Here's how the part is built. I have some questions about the finished solid (model axes, mm). Face numbers are marked on the shaded views. A direction names the side the tool comes from. Give positions to 0.01 mm unless a question says otherwise; leave off trailing zeros. Loops run counter-clockwise (first coordinate to the right, second up) from the corner with the lowest first, then second, coordinate; pieces in that order, holes last.
Q1. I'm going to push a flat-ended pin straight in: P1, Ø8.5, axis at x = 23.65, z = -10, coming from the +Y side. Where does the tip first touch, or does it pass through?
Q2. Thinking about a two-plate mould opening in X: for the marked faces 1, 2 and 3, which applies, pulls with the +X half, pulls with the -X half, needs draft (parallel to the pull), parting line crosses it, or undercut?
Q3. For the marked faces 4 and 5, which set-ups out of +Z, -Z, +X, -X, +Y, -Y let a thin tool reach every point of the face, with its end or its side?
Q4. Suppose I cut it at B-B (y = 7.5). List the corners of the cut face in (x, z) for me, and give its area (3 significant figures).
Q5. I need wall thicknesses on probe 1 along X at (y, z) = (3.75, -35); probe 2 along Z at (x, y) = (56, 3.75); probe 3 along Z at (x, y) = (23.65, 5.5). Which ranges of each line are inside material? Lowest first, please.
Q6. Suppose I cut it at A-A (z = -39). List the corners of the cut face in (x, y) for me.
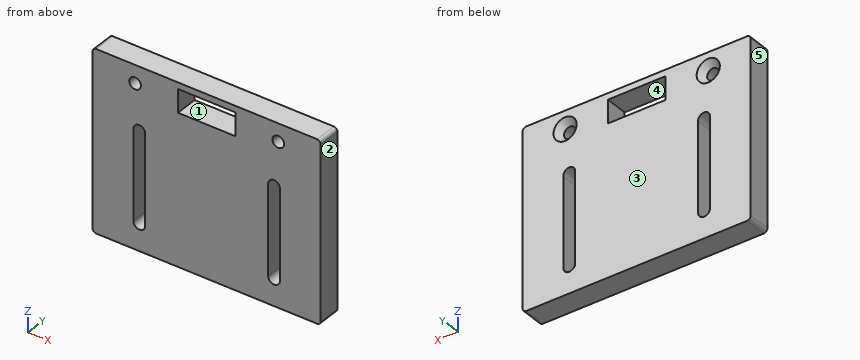
```python
from build123d import *

# Parameters (mm, degrees)
SKETCH1_W                                        = 127
SKETCH1_H                                        = 100
BOSS_EXTRUDE1_DEPTH                              = 12.7
CUT_EXTRUDE1_DEPTH                               = 12.7
CUT_EXTRUDE2_DEPTH                               = 163.142807426
FILLET1_R                                        = 2
CSK_FOR_1_4_FLAT_HEAD_MACHINE_SCREW1_D           = 6.5278
CSK_FOR_1_4_FLAT_HEAD_MACHINE_SCREW1_CSINK_D     = 12.8778
CSK_FOR_1_4_FLAT_HEAD_MACHINE_SCREW1_CSINK_ANGLE = 82


with BuildPart() as part:
    # Sketch1 → Boss-Extrude1 (new body)
    with BuildSketch(Plane(origin=(0, 0, 0), x_dir=(1, 0, 0), z_dir=(0, 1, 0))):
        with Locations((63.5, 50)):
            Rectangle(SKETCH1_W, SKETCH1_H)
    extrude(amount=BOSS_EXTRUDE1_DEPTH)

    # Sketch2 → Cut-Extrude1 (cut)
    with BuildSketch(Plane(origin=(0, 12.7, 0), x_dir=(1, 0, 0), z_dir=(0, 1, 0))):
        Polygon((47.53, 10), (47.53, 16.45), (79.48, 16.45), (79.48, 10), (79.48, 3.55), (47.53, 3.55), align=None)
    extrude(amount=-CUT_EXTRUDE1_DEPTH, mode=Mode.SUBTRACT)

    # Sketch6 → Cut-Extrude2 (cut, through all)
    with BuildSketch(Plane(origin=(0, 12.7, 0), x_dir=(1, 0, 0), z_dir=(0, 1, 0))):
        with BuildLine():
            Line((22.690847092, 35), (22.690847092, 85))
            ThreePointArc((22.690847092, 85), (25.990847092, 88.3), (29.290847092, 85))
            Line((29.290847092, 85), (29.290847092, 35))
            ThreePointArc((29.290847092, 35), (25.990847092, 31.7), (22.690847092, 35))
        make_face()
        with BuildLine():
            Line((97.720847092, 35.000004619), (97.720847092, 84.999995381))
            ThreePointArc((97.720847092, 84.999995381), (100.881876157, 88.297072501), (104.30914268, 85.2776907))
            Line((104.30914268, 85.2776907), (104.30914268, 35.2776907))
            ThreePointArc((104.30914268, 35.2776907), (101.159813412, 31.702927304), (97.720847092, 35.000004619))
        make_face()
    extrude(amount=-CUT_EXTRUDE2_DEPTH, mode=Mode.SUBTRACT)

    # Fillet1
    fillet1_edges = [part.edges().sort_by_distance(p)[0] for p in [
        (0, 6.35, -100),
        (127, 6.35, -100),
        (127, 6.35, 0),
        (0, 6.35, 0),
    ]]
    fillet(fillet1_edges, radius=FILLET1_R)

    # CSK for 1/4 Flat Head Machine Screw1 (through all)
    with Locations(Plane(origin=(23.65, 12.7, -9.996892397), x_dir=(0, 0, 1), z_dir=(0, 1, 0))):
        with Locations((0, 0), (0, 79.7)):
            CounterSinkHole(CSK_FOR_1_4_FLAT_HEAD_MACHINE_SCREW1_D / 2, CSK_FOR_1_4_FLAT_HEAD_MACHINE_SCREW1_CSINK_D / 2, counter_sink_angle=CSK_FOR_1_4_FLAT_HEAD_MACHINE_SCREW1_CSINK_ANGLE)


solid = part.part
```
Solutions:
1. P1: stops at y = 10.19
2. face 1: undercut
2. face 2: pulls with the +X half
2. face 3: needs draft
3. face 4: +Y, -Y
3. face 5: +Z, -Z, -X, +Y, -Y
4. outline: (0, -98) arc R2 ccw to (2, -100) - (125, -100) arc R2 ccw to (127, -98) - (127, -2) arc R2 ccw to (125, 0) - (2, 0) arc R2 ccw to (0, -2) - close; hole circle Ø6.53 at (23.65, -10); hole (22.69, -85) arc R3.3 ccw to (29.29, -85) - (29.29, -35) arc R3.3 ccw to (22.69, -35) - close; hole (47.53, -16.45) - (79.48, -16.45) - (79.48, -3.55) - (47.53, -3.55) - close; hole (97.72, -85) arc R3.3 ccw to (104.31, -85.28) - (104.31, -35.28) arc R3.3 ccw (long way) to (97.72, -35) - close; hole circle Ø6.53 at (103.35, -10)
4. area: 11,500 mm2
5. probe 1: x = 0 to 22.69, 29.29 to 97.72, 104.32 to 127
5. probe 2: z = -100 to -16.45, -3.55 to 0
5. probe 3: z = -100 to -87.33, -32.67 to -13.26, -6.73 to 0
6. outline: (0, 0) - (22.69, 0) - (22.69, 12.7) - (0, 12.7) - close; (29.29, 0) - (97.72, 0) - (97.72, 12.7) - (29.29, 12.7) - close; (104.31, 0) - (127, 0) - (127, 12.7) - (104.31, 12.7) - close
